from build123d import *

# Parameters (mm, degrees)
SKETCH1_W           = 28.32
SKETCH1_H           = 23.24
SKETCH1_R           = 2.3
SKETCH1_W_2         = 14.72
SKETCH1_H_2         = 4.6
BOSS_EXTRUDE1_DEPTH = 2
SKETCH1_3_R         = 2.3
SKETCH1_3_R_2       = 1.3
BOSS_EXTRUDE2_DEPTH = 4
SKETCH1_4_W         = 30.32
SKETCH1_4_H         = 33.24
SKETCH1_4_W_2       = 28.32
SKETCH1_4_H_2       = 23.24
SKETCH1_4_R         = 2.1
BOSS_EXTRUDE3_DEPTH = 8
FILLET2_R           = 2


with BuildPart() as part:
    # Sketch1 → Boss-Extrude1 (new body)
    with BuildSketch(Plane(origin=(0, 0, 0), x_dir=(1, 0, 0), z_dir=(0, 1, 0))):
        Rectangle(SKETCH1_W, SKETCH1_H)
        with Locations(Location((10.16, -7.62, 0), (0, 0, 270))):
            Circle(SKETCH1_R, mode=Mode.SUBTRACT)
        with Locations(Location((10.16, 7.62, 0), (0, 0, 270))):
            Circle(SKETCH1_R, mode=Mode.SUBTRACT)
        with Locations(Location((-10.16, -7.62, 0), (0, 0, 270))):
            Circle(SKETCH1_R, mode=Mode.SUBTRACT)
        with Locations(Location((-10.16, 7.62, 0), (0, 0, 270))):
            Circle(SKETCH1_R, mode=Mode.SUBTRACT)
        with Locations((0, -7.62)):
            Rectangle(SKETCH1_W_2, SKETCH1_H_2, mode=Mode.SUBTRACT)
    extrude(amount=BOSS_EXTRUDE1_DEPTH)

    # Sketch1_3 → Boss-Extrude2 (add)
    # profile 1 of 4: a face of its own
    with BuildSketch(Plane(origin=(0, 0, 0), x_dir=(1, 0, 0), z_dir=(0, 1, 0))):
        with Locations(Location((-10.16, -7.62, 0), (0, 0, 270))):
            Circle(SKETCH1_3_R)
        with Locations(Location((-10.16, -7.62, 0), (0, 0, 270))):
            Circle(SKETCH1_3_R_2, mode=Mode.SUBTRACT)
    # profile 2 of 4: a face of its own
    with BuildSketch(Plane(origin=(0, 0, 0), x_dir=(1, 0, 0), z_dir=(0, 1, 0))):
        with Locations(Location((10.16, -7.62, 0), (0, 0, 270))):
            Circle(SKETCH1_3_R)
        with Locations(Location((10.16, -7.62, 0), (0, 0, 270))):
            Circle(SKETCH1_3_R_2, mode=Mode.SUBTRACT)
    # profile 3 of 4: a face of its own
    with BuildSketch(Plane(origin=(0, 0, 0), x_dir=(1, 0, 0), z_dir=(0, 1, 0))):
        with Locations(Location((10.16, 7.62, 0), (0, 0, 270))):
            Circle(SKETCH1_3_R)
        with Locations(Location((10.16, 7.62, 0), (0, 0, 270))):
            Circle(SKETCH1_3_R_2, mode=Mode.SUBTRACT)
    # profile 4 of 4: a face of its own
    with BuildSketch(Plane(origin=(0, 0, 0), x_dir=(1, 0, 0), z_dir=(0, 1, 0))):
        with Locations(Location((-10.16, 7.62, 0), (0, 0, 270))):
            Circle(SKETCH1_3_R)
        with Locations(Location((-10.16, 7.62, 0), (0, 0, 270))):
            Circle(SKETCH1_3_R_2, mode=Mode.SUBTRACT)
    extrude(amount=BOSS_EXTRUDE2_DEPTH)

    # Sketch1_4 → Boss-Extrude3 (add)
    with BuildSketch(Plane(origin=(0, 0, 0), x_dir=(1, 0, 0), z_dir=(0, 1, 0))):
        with Locations((0, -4)):
            Rectangle(SKETCH1_4_W, SKETCH1_4_H)
        Rectangle(SKETCH1_4_W_2, SKETCH1_4_H_2, mode=Mode.SUBTRACT)
        with Locations(Location((12, -16.62, 0), (0, 0, 270))):
            Circle(SKETCH1_4_R, mode=Mode.SUBTRACT)
        with Locations(Location((-12, -16.62, 0), (0, 0, 270))):
            Circle(SKETCH1_4_R, mode=Mode.SUBTRACT)
        with Locations(Location((-4, -16.62, 0), (0, 0, 270))):
            Circle(SKETCH1_4_R, mode=Mode.SUBTRACT)
        with Locations(Location((4, -16.62, 0), (0, 0, 270))):
            Circle(SKETCH1_4_R, mode=Mode.SUBTRACT)
    extrude(amount=BOSS_EXTRUDE3_DEPTH)

    # Fillet2
    fillet2_edges = [part.edges().sort_by_distance(p)[0] for p in [
        (-15.16, 4, 20.62),
        (15.16, 4, 20.62),
        (15.16, 4, -12.62),
        (-15.16, 4, -12.62),
    ]]
    fillet(fillet2_edges, radius=FILLET2_R)


solid = part.part
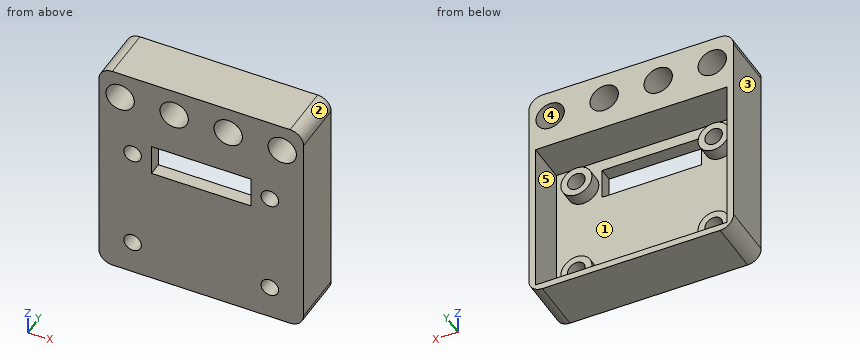
Here's how the part is built. I have some questions about the finished solid (model axes, mm). Face numbers are marked on the shaded views. A direction names the side the tool comes from. Round coordinates to 2 decimals unless told otherwise and drop trailing zeros. Order: outer loops, then holes, each group sorted by start corner. A loop starts at its lowest first (then second) coordinate and runs counter-clockwise, first axis right, second up. Notation, with made-up numbers: (9.25, 15) -> (33.25, 15) arc R13 ccw to (33.25, 22) -> close; hole circle Ø9 at (-4, -22.5). An arc over 180 degrees is marked (long way). Return JSON: item names as keys, results as strings.
Q1. For pin 1 Ø4 at (x, z) = (10.16, -7.62) entering from -Y; pin 2 Ø3 at (x, z) = (-10.16, -7.62) entering from +Y; pin 3 Ø2 at (x, z) = (-1, 6) entering from +Y, each with a flat end and sliding along its axis, tell me the tip position at first contact or that it passes through.
Filled sheet:
{"pin 1": "stops at y = 0", "pin 2": "stops at y = 4", "pin 3": "stops at y = 2"}
Q2. I need wall thicknesses on line 1 along X through (y, z) = (5.25, 16.62); line 2 along X through (y, z) = (6, 18); line 3 along X through (y, z) = (5.75, 10). Which ranges of each line are inside material? Lowest first, please. Write a range as from..to.
Filled sheet:
{"line 1": "x = -15.16..-14.1, -9.9..-6.1, -1.9..1.9, 6.1..9.9, 14.1..15.16", "line 2": "x = -15.16..-13.58, -10.42..-5.58, -2.42..2.42, 5.58..10.42, 13.58..15.16", "line 3": "x = -15.16..-14.16, 14.16..15.16"}
Q3. Which directions (+Z, -Z, +X, -X, +Y, -Y) give clear straight access to the entire face, cutting with the end or side of a thin tool? Please do the marked faces 4 and 5.
Filled sheet:
{"face 4": "+Y, -Y", "face 5": "+Y"}
Q4. If we section it at C-C on x = -12: List the corners of the cut face in (y, z) for me, plus the area to 3 significant figures.
Filled sheet:
{"outline": "(0, -12.62) -> (8, -12.62) -> (8, -11.62) -> (2, -11.62) -> (2, -9) -> (4, -9) -> (4, -6.24) -> (2, -6.24) -> (2, 6.24) -> (4, 6.24) -> (4, 9) -> (2, 9) -> (2, 11.62) -> (8, 11.62) -> (8, 14.52) -> (0, 14.52) -> close; (0, 18.72) -> (8, 18.72) -> (8, 20.62) -> (0, 20.62) -> close", "area": "104 mm^2"}
Q5. If we section it at D-D on y = 6: List the corners of the cut face in (x, z) for me, plus the area to 3 significant figures.
Filled sheet:
{"outline": "(-15.16, -10.62) arc R2 ccw to (-13.16, -12.62) -> (13.16, -12.62) arc R2 ccw to (15.16, -10.62) -> (15.16, 18.62) arc R2 ccw to (13.16, 20.62) -> (-13.16, 20.62) arc R2 ccw to (-15.16, 18.62) -> close; hole (-14.16, -11.62) -> (14.16, -11.62) -> (14.16, 11.62) -> (-14.16, 11.62) -> close; hole circle Ø4.2 at (-12, 16.62); hole circle Ø4.2 at (-4, 16.62); hole circle Ø4.2 at (4, 16.62); hole circle Ø4.2 at (12, 16.62)", "area": "291 mm^2"}
Q6. If we section it at A-A on z = -7.62: List the corners of the cut face in (x, y) for me.
Filled sheet:
{"outline": "(-15.16, 0) -> (-11.46, 0) -> (-11.46, 4) -> (-12.46, 4) -> (-12.46, 2) -> (-14.16, 2) -> (-14.16, 8) -> (-15.16, 8) -> close; (-8.86, 0) -> (8.86, 0) -> (8.86, 4) -> (7.86, 4) -> (7.86, 2) -> (-7.86, 2) -> (-7.86, 4) -> (-8.86, 4) -> close; (11.46, 0) -> (15.16, 0) -> (15.16, 8) -> (14.16, 8) -> (14.16, 2) -> (12.46, 2) -> (12.46, 4) -> (11.46, 4) -> close"}
Q7. If we section it at B-B on z = 7.62: List the corners of the cut face in (x, y) for me, plus the area to 3 significant figures.
Filled sheet:
{"outline": "(-15.16, 0) -> (-11.46, 0) -> (-11.46, 4) -> (-12.46, 4) -> (-12.46, 2) -> (-14.16, 2) -> (-14.16, 8) -> (-15.16, 8) -> close; (-8.86, 0) -> (-7.36, 0) -> (-7.36, 2) -> (-7.86, 2) -> (-7.86, 4) -> (-8.86, 4) -> close; (7.36, 0) -> (8.86, 0) -> (8.86, 4) -> (7.86, 4) -> (7.86, 2) -> (7.36, 2) -> close; (11.46, 0) -> (15.16, 0) -> (15.16, 8) -> (14.16, 8) -> (14.16, 2) -> (12.46, 2) -> (12.46, 4) -> (11.46, 4) -> close", "area": "40.8 mm^2"}
Q8. If we mould it in two halves opening along Z, with no side actions, what happens to the marked faces 1, 2 and 3? For each: released by +Z, released by -Z, zero draft, split by the parting line, or undercut.
Filled sheet:
{"face 1": "undercut", "face 2": "released by +Z", "face 3": "zero draft"}
